Autodesk Inventor part; units mm, degrees
ref_plane "YZ Plane" through (0, 0, 0) normal (1, 0, 0) x (0, 1, 0)
ref_plane "XZ Plane" through (0, 0, 0) normal (0, 1, 0) x (-1, 0, 0)
ref_plane "XY Plane" through (0, 0, 0) normal (0, 0, 1) x (1, 0, 0)
sketch "Sketch1" plane through (0, 0, 0) normal (0, 0, 1) x (1, 0, 0)
  line L0 (0, 0) -> (-350, 0)
  line L1 (0, -100) -> (0, 0)
  line L2 (-350, 0) -> (-350, -80)
  line L3 (-350, -80) -> (0, -100)
  point P0 (0, -50)
  dimension "d32" = 100
  dimension "d60" = 80
  dimension "d61" = 350
extrude "Plate1" add sketch "Sketch1" along normal blind 2
sketch "Sketch8" plane through (0, 0, 2) normal (0, 0, 1) x (1, 0, 0)
  line L0 (-29.75, -58.25) -> (-60.25, -58.25)
  line L1 (-60.25, -58.25) -> (-60.25, -27.75)
  line L2 (-60.25, -27.75) -> (-29.75, -27.75)
  line L3 (-29.75, -27.75) -> (-29.75, -58.25)
  line L4 (-29.75, -58.25) -> (-60.25, -27.75) construction
  line L5 (-60.25, -58.25) -> (-29.75, -27.75) construction
  circle A0 centre (-18.4835, -69.5165) radius 2.5
  circle A1 centre (-71.5165, -69.5165) radius 2.5
  circle A2 centre (-71.5165, -16.4835) radius 2.5
  circle A3 centre (-18.4835, -16.4835) radius 2.5
  circle A4 centre (-45, -43) radius 37.5 construction
  line L6 (0, 0) -> (0, -100)
  line L7 (-350, 0) -> (0, 0)
  line L8 (-60.25, -58.25) -> (-71.5165, -69.5165) construction
  dimension "d51" = 30.5
  dimension "d52" = 30.5
  dimension "d53" = 5
  dimension "d72" = 45
  dimension "d73" = 43
  dimension "d74" = 15.9332
  dimension "d75" = 75
extrude "Cut3" cut sketch "Sketch8" against normal blind 2
pattern_linear "Rectangular Pattern1" count 3 spacing 120 along (-1, 0, 0) of "Cut3"
sketch "Sketch9" plane through (0, -2, 2) normal (0, 1, 0) x (-1, 0, 0)
  line L0 (350, 0) -> (0, 0)
  line L1 (0, 0) -> (0, -64)
  line L2 (0, -64) -> (350, -64)
  line L3 (350, -64) -> (350, 0)
edge flange "Flange3" height 64 angle 90 thickness 2 bend radius 2.75 thickness toward (0, 1, 0) relief round relief width 2 relief depth 1 edges at (-175, 0, 0) wall of the first edge with corners at (-350, -2, 2) (0, -2, 2) (0, -2, -62) (-350, -2, -62)
bend "Bend3"
corner "Corner3"
equation "\"d32\" = Main_way_hight"
equation "\"d51\" = d52"
equation "\"d55\" = Thickness"
equation "\"d2\" = Thickness"
equation "\"d62\" = BendReliefWidth"
equation "\"d63\" = BendReliefDepth"
equation "\"d64\" = MinimumRemnant"
equation "\"d65\" = TransitionRadius"
equation "\"d66\" = MAIN_7_central_window_width + 2 * Thickness"
equation "\"d68\" = BendRadius"
equation "\"d69\" = CornerReliefSize"
equation "\"d70\" = GapSize"
equation "\"d71\" = JacobiRadiusSize"
equation "\"BendReliefWidth\" = Thickness"
equation "\"BendReliefDepth\" = 0.5 * Thickness"
equation "\"CornerReliefSize\" = 4 * Thickness"
equation "\"MinimumRemnant\" = 2 * Thickness"
equation "\"TransitionRadius\" = BendRadius"
equation "\"JacobiRadiusSize\" = BendRadius"
equation "\"GapSize\" = Thickness"
equation "\"Main_way_hight\" = 100"
properties part number "ANP 1422 BOTTOM FDS diameter way up" material "Stainless Steel"
Part model, mm, in its own coordinate system. A direction names the side the tool comes from. Round coordinates to 2 decimals unless told otherwise and drop trailing zeros. Loops run counter-clockwise (first coordinate to the right, second up) from the corner with the lowest first, then second, coordinate; pieces in that order, holes last.
Item 1: Cut at C-C, the plane z = -12.5. Give the cut face in (x, y).
Item 2: 3-axis set-ups, long thin cutter, end or side, ignore diameter. For faces 1 (the face through (-350, -22, 1)), 2 (the face through (-173, -2, -32)): which of +Z, -Z, +X, -X, +Y, -Y reach the whole face in a straight line?
Item 3: Drill centre lines: line 1 (Z direction, x = -214.5, y = -67); line 2 (Y direction, x = -40, z = -35); line 3 (Y direction, x = -114, z = -1.5). Where is each one in solid material? Low to high.
Item 4: Cut at D-D, the plane y = -90. Give the cut face in (x, z).
Item 5: Drop flat-ended pins along their axis: P1, Ø1.6, axis at x = -40, z = 0.5, coming from the +Y side; P2, Ø1, axis at x = -287.5, z = 1.5, coming from the +Y side; P3, Ø1, axis at x = -50.5, z = 1, coming from the -Y side. Give the stop position or say it passes through.
Item 6: Cut at A-A, the plane y = -44.5. Give the cut face in (x, z).
Item 7: Cut at B-B, the plane x = -84. Give the cut face in (y, z), then the cut area to 3 significant figures.
A:
1. outline: (-350, -2) - (0, -2) - (0, 0) - (-350, 0) - close
2. face 1: +Z, -Z, -X, +Y, -Y
2. face 2: -Z, +X, -X, -Y
3. line 1: z = 0 to 2
3. line 2: y = -2 to 0
3. line 3: y = -2.3 to -0.17
4. outline: (-175, 0) - (0, 0) - (0, 2) - (-175, 2) - close
5. P1: stops at y = -0.68
5. P2: stops at y = -1.83
5. P3: stops at y = -97.14
6. outline: (-350, 0) - (-300.25, 0) - (-300.25, 2) - (-350, 2) - close; (-269.75, 0) - (-180.25, 0) - (-180.25, 2) - (-269.75, 2) - close; (-149.75, 0) - (-60.25, 0) - (-60.25, 2) - (-149.75, 2) - close; (-29.75, 0) - (0, 0) - (0, 2) - (-29.75, 2) - close
7. outline: (-95.2, 0) - (-4.75, 0) arc R2.75 cw to (-2, -2.75) - (-2, -62) - (0, -62) - (0, -2.75) arc R4.75 ccw to (-4.75, 2) - (-95.2, 2) - close
7. area: 311 mm2
